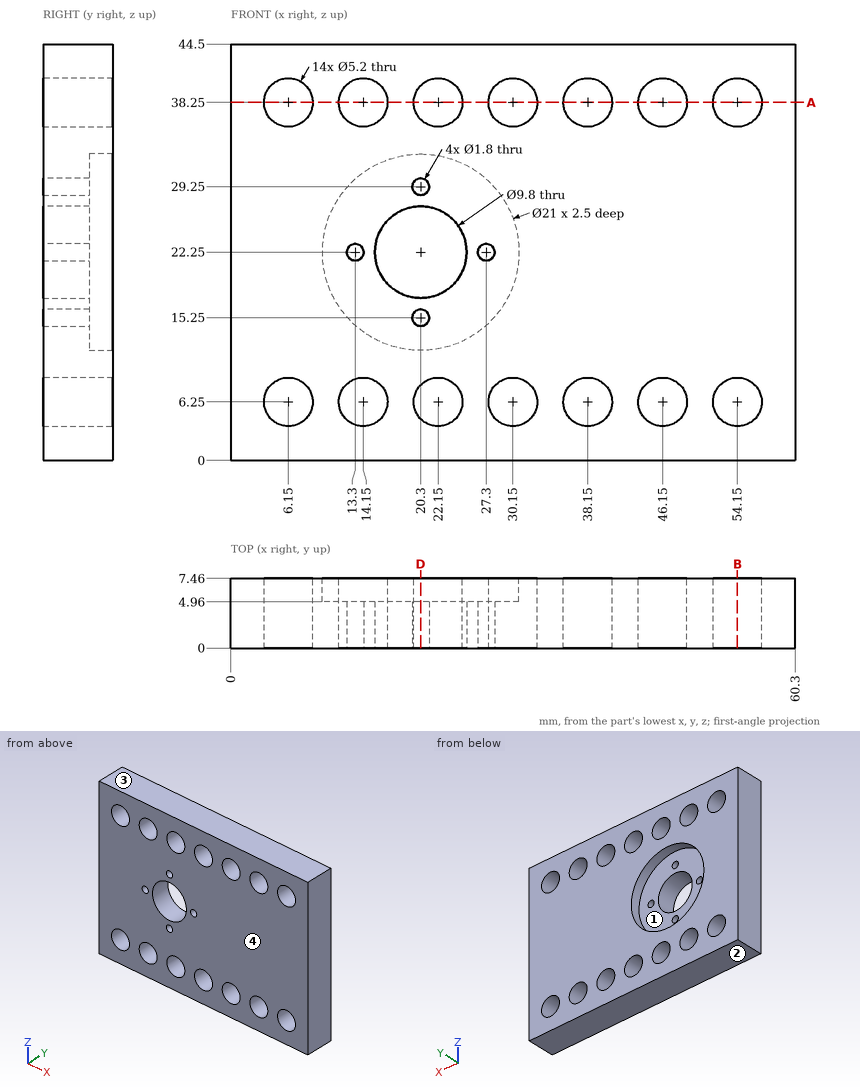
The figure shows three views and two pictorial views of one solid part (mm, origin at its lowest corner). Answer the questions. Round coordinates to 2 decimals unless told otherwise and drop trailing zeros. Loops run counter-clockwise (first coordinate to the right, second up) from the corner with the lowest first, then second, coordinate; pieces in that order, holes last. Notation, with made-up numbers: M -29,-35 L 5,-35 A14 ccw 5,-28 Z; hole C -21,43.25 d5. An arc over 180 degrees is marked long. Write each question's results on one line, items separated by ' | '. Start each with the question number.
1) Determine the mould class of the marked faces 1, 2, 3 and 4 for opening direction Z: pulls with the +Z half, pulls with the -Z half, needs draft (parallel to the pull), parting line crosses it, or undercut.
2) Each of these flat-tipped pins is pushed along its axis until it touches: pin 1 (4.5 mm diameter, centred on x = 38.15, z = 6.25, fed in from -Y); pin 2 (8.5 mm diameter, centred on x = 14.15, z = 38.25, fed in from -Y); pin 3 (10.5 mm diameter, centred on x = 15.5, z = 23, fed in from +Y). Where does it stop, or does it pass through?
3) Straight lines are drawn through the part: probe 1 along X at (y, z) = (6.2, 22.25); probe 2 along X at (y, z) = (1.25, 22); probe 3 along Z at (x, y) = (24, 4.5). For each, find the intervals that lie inside material, in ascending order.
4) Find section B-B on x = 54.15. Write down the section's boundary in (y, z).
5) Find section D-D on x = 20.3. Write down the section's boundary in (y, z), plus the area to 3 significant figures.
6) Find section A-A on z = 38.25. Count the separate pieces of the cut face and the enclosed holes in it, plus the area to 3 significant figures.
Final values:
1) face 1: undercut | face 2: pulls with the -Z half | face 3: pulls with the +Z half | face 4: needs draft
2) pin 1: through | pin 2: y = 0 | pin 3: y = 4.96
3) probe 1: 0 to 9.8, 30.8 to 60.3 | probe 2: 0 to 12.44, 14.16 to 15.41, 25.19 to 26.44, 28.16 to 60.3 | probe 3: 0 to 4.42, 8.08 to 19.04, 25.46 to 36.42, 40.08 to 44.5
4) outline: M 0,0 L 7.46,0 L 7.46,3.65 L 0,3.65 Z; M 0,8.85 L 7.46,8.85 L 7.46,35.65 L 0,35.65 Z; M 0,40.85 L 7.46,40.85 L 7.46,44.5 L 0,44.5 Z
5) outline: M 0,0 L 7.46,0 L 7.46,4.42 L 0,4.42 Z; M 0,8.08 L 7.46,8.08 L 7.46,11.75 L 4.96,11.75 L 4.96,14.35 L 0,14.35 Z; M 0,16.15 L 4.96,16.15 L 4.96,17.35 L 0,17.35 Z; M 0,27.15 L 4.96,27.15 L 4.96,28.35 L 0,28.35 Z; M 0,30.15 L 4.96,30.15 L 4.96,32.75 L 7.46,32.75 L 7.46,36.42 L 0,36.42 Z; M 0,40.08 L 7.46,40.08 L 7.46,44.5 L 0,44.5 Z | area: 158 mm²
6) separate pieces: 8 | enclosed holes: 0 | area: 178 mm²
